```python
from build123d import *

# Parameters (mm, degrees)
SZKIC1_W                    = 10
SZKIC1_H                    = 10
DODANIE_WYCI_GNI_CIE1_DEPTH = 200
SZKIC2_R                    = 1
WYTNIJ_WYCI_GNI_CIE1_DEPTH  = 10
WYTNIJ_WYCI_GNI_CIE2_START  = -10
SZKIC3_R                    = 1
WYTNIJ_WYCI_GNI_CIE2_DEPTH  = 10
SZKIC4_W                    = 10
SZKIC4_H                    = 3
DODANIE_WYCI_GNI_CIE2_DEPTH = 3
SZKIC6_W                    = 10
SZKIC6_H                    = 3
DODANIE_WYCI_GNI_CIE3_DEPTH = 3


with BuildPart() as part:
    # Szkic1 → Dodanie-wyciągnięcie1 (new body)
    with BuildSketch(Plane(origin=(0, 0, 0), x_dir=(1, 0, 0), z_dir=(0, 1, 0))):
        Rectangle(SZKIC1_W, SZKIC1_H)
    extrude(amount=DODANIE_WYCI_GNI_CIE1_DEPTH)

    # Szkic2 → Wytnij-wyciągnięcie1 (cut)
    with BuildSketch(Plane(origin=(0, 200, 0), x_dir=(1, 0, 0), z_dir=(0, 1, 0))):
        with Locations(Location((0, 0, 0), (0, 0, 270))):
            Circle(SZKIC2_R)
    extrude(amount=-WYTNIJ_WYCI_GNI_CIE1_DEPTH, mode=Mode.SUBTRACT)

    # Szkic3 → Wytnij-wyciągnięcie2 (cut)
    with BuildSketch(Plane.XZ.offset(WYTNIJ_WYCI_GNI_CIE2_START)):
        with Locations(Location((0, 0, 0), (0, 0, 90))):
            Circle(SZKIC3_R)
    extrude(amount=WYTNIJ_WYCI_GNI_CIE2_DEPTH, mode=Mode.SUBTRACT)

    # Szkic4 → Dodanie-wyciągnięcie2 (add)
    with BuildSketch(Plane.XY.offset(5)):
        with Locations((0, 71.5)):
            Rectangle(SZKIC4_W, SZKIC4_H)
        with Locations((0, 78.5)):
            Rectangle(SZKIC4_W, SZKIC4_H)
    extrude(amount=DODANIE_WYCI_GNI_CIE2_DEPTH)

    # Szkic6 → Dodanie-wyciągnięcie3 (add)
    with BuildSketch(Plane(origin=(5, 0, 0), x_dir=(0, 0, -1), z_dir=(1, 0, 0))):
        with Locations((0, 71.5)):
            Rectangle(SZKIC6_W, SZKIC6_H)
        with Locations((0, 78.5)):
            Rectangle(SZKIC6_W, SZKIC6_H)
    extrude(amount=DODANIE_WYCI_GNI_CIE3_DEPTH)


solid = part.part
```
Part model, mm, in its own coordinate system. A direction names the side the tool comes from. Round coordinates to 2 decimals unless told otherwise and drop trailing zeros. Write each loop counter-clockwise with the first axis right and the second up, starting at its lowest first coordinate (ties: lowest second). Pieces come first, ordered by that corner, then holes.
Item 1: Drop flat-ended pins along their axis: pin 1 Ø1.5 at (x, z) = (7, -0.5) entering from -Y; pin 2 Ø1.5 at (x, z) = (6, -1.5) entering from +Y; pin 3 Ø0.6 at (x, z) = (0.5, 0) entering from -Y; pin 4 Ø3.5 at (x, z) = (6.5, -1.5) entering from +Y. Give the stop position or say it passes through.
Results:
pin 1: stops at y = 70
pin 2: stops at y = 80
pin 3: stops at y = 10
pin 4: stops at y = 200
Item 2: Probe L1, parallel to Y at x = 6, z = 0.25; L2, parallel to X at y = 6, z = 0; L3, parallel to Z at x = 1.75, y = 107.5. List the from-to ranges inside material, lowest first.
Results:
L1: y = 70 to 73, 77 to 80
L2: x = -5 to -1, 1 to 5
L3: z = -5 to 5
Item 3: Which spindle directions (+Z, -Z, +X, -X, +Y, -Y) get a long thin tool onto all of the face, cutting with end or side? Do faces 1 (the flat face through (0, 139, 5)), 2 (the flat face through (5, 75, 0)), 3 (the flat face through (0, 35, 5)), 4 (the flat face through (5, 35, 0)). Say none if no direction does.
Results:
face 1: +Z, +X, -X, +Y
face 2: +Z, -Z, +X
face 3: +Z, +X, -X, -Y
face 4: +Z, -Z, +X, -Y
Item 4: Two-plate mould, pull along Y, no slides. Class faces 5 (the flat face through (5, 139, 0)), 6 (the flat face through (0, 75, 5)), 7 (the flat face through (-0.1, 0, -1.2)): +Y half, -Y half, draft (parallel to the pull), parting line (faces both ways), or undercut.
Results:
face 5: draft
face 6: undercut
face 7: -Y half
Item 5: Cut at A-A, the plane y = 184.5. Give the cut face in (x, z), plus the area to 3 significant figures.
Results:
outline: (-5, -5) - (5, -5) - (5, 5) - (-5, 5) - close
area: 100 mm2
